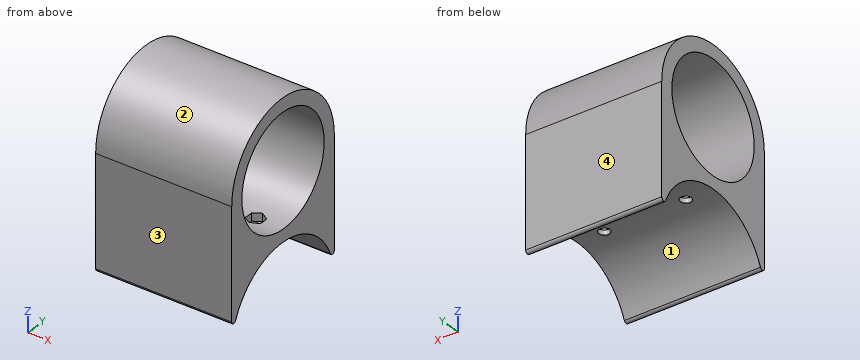
```python
from build123d import *

# Parameters (mm, degrees)
EXTRUDE_1_DEPTH      = 25
EXTRUDE_1_DEPTH_BACK = 25
SKETCH_1_R           = 20.25
SKETCH_2_R           = 2
CUT_EXTRUDE_1_DEPTH  = 41
CUT_EXTRUDE_2_DEPTH  = 3


with BuildPart() as part:
    # 草图1 → 凸台-拉伸1 (new, two sides: drawn at the far end of the back side and taken through both)
    with BuildSketch(Plane(origin=(0, 0, 0), x_dir=(0, 0, -1), z_dir=(1, 0, 0)).offset(-EXTRUDE_1_DEPTH_BACK)):
        with BuildLine():
            Line((39.950124379, 25.25), (0, 25.25))
            ThreePointArc((0, 25.25), (-25.25, 0), (0, -25.25))
            Line((0, -25.25), (39.950124379, -25.25))
            ThreePointArc((39.950124379, -25.25), (40.930891814, -24.445180015), (40.332976783, -23.326190476))
            ThreePointArc((40.332976783, -23.326190476), (24.75, 0), (40.332976783, 23.326190476))
            ThreePointArc((40.332976783, 23.326190476), (40.930891814, 24.445180015), (39.950124379, 25.25))
        make_face()
        Circle(SKETCH_1_R, mode=Mode.SUBTRACT)
    extrude(amount=EXTRUDE_1_DEPTH + EXTRUDE_1_DEPTH_BACK)

    # 草图2 → 切除-拉伸1 (cut)
    with BuildSketch(Plane.XY):
        with Locations((-15, 0)):
            Circle(SKETCH_2_R)
        with Locations((15, 0)):
            Circle(SKETCH_2_R)
    extrude(amount=-CUT_EXTRUDE_1_DEPTH, mode=Mode.SUBTRACT)

    # 草图3 → 切除-拉伸2 (cut)
    with BuildSketch(Plane.XY.offset(-20)):
        Polygon((-15, 3.25), (-17.814582562, 1.625), (-17.814582562, -1.625), (-15, -3.25), (-12.185417438, -1.625), (-12.185417438, 1.625), align=None)
        Polygon((15, 3.25), (12.185417438, 1.625), (12.185417438, -1.625), (15, -3.25), (17.814582562, -1.625), (17.814582562, 1.625), align=None)
    extrude(amount=-CUT_EXTRUDE_2_DEPTH, mode=Mode.SUBTRACT)


solid = part.part
```
Verification items for the finished model (mm, model axes). Face numbers are marked on the shaded views. Round coordinates to 2 decimals unless told otherwise and drop trailing zeros. Order: outer loops, then holes, each group sorted by start corner. A loop starts at its lowest first (then second) coordinate and runs counter-clockwise, first axis right, second up. Notation, with made-up numbers: (11.5, 16) - (48.5, 16) arc R22 ccw to (48.5, 46) - close; hole circle Ø6 at (17.5, 48.25). An arc over 180 degrees is marked (long way). Use CSV: the item, a comma, the result in double quotes.
(1) Thickness scan on probe 1 along X at (y, z) = (0, -23.45); probe 2 along Y at (x, z) = (-15, -24); probe 3 along Y at (x, z) = (13, 0). Record the ranges inside material, lowest first. Write a range as from..to.
Entries:
probe 1,"-25..-17, -13..13, 17..25"
probe 2,"-25.25..-2, 2..25.25"
probe 3,"-25.25..-20.25, 20.25..25.25"
(2) Section check B-B on y = 0. Record the boundary of the cut face in (x, z).
Entries:
outline,"(-25, -24.75) - (-17, -24.75) - (-17, -23) - (-17.81, -23) - (-17.81, -20.25) - (-25, -20.25) - close; (-25, 20.25) - (25, 20.25) - (25, 25.25) - (-25, 25.25) - close; (-13, -24.75) - (13, -24.75) - (13, -23) - (12.19, -23) - (12.19, -20.25) - (-12.19, -20.25) - (-12.19, -23) - (-13, -23) - close; (17, -24.75) - (25, -24.75) - (25, -20.25) - (17.81, -20.25) - (17.81, -23) - (17, -23) - close"
(3) Section check D-D on y = 11. Record the boundary of the cut face in (x, z).
Entries:
outline,"(-25, -27.27) - (25, -27.27) - (25, -17) - (-25, -17) - close; (-25, 17) - (25, 17) - (25, 22.73) - (-25, 22.73) - close"
(4) Gauge pin test, flat ends, axial feed: pin 1 Ø1.5 at (x, y) = (-4.5, -17.5) entering from +Z; pin 2 Ø3 at (x, y) = (-15, 0.5) entering from +Z; pin 3 Ø3 at (x, y) = (15.5, 19.5) entering from +Z. Record the tip position at first contact, or that the pin passes through.
Entries:
pin 1,"z = 18.89"
pin 2,"z = 25.25"
pin 3,"z = 17.71"
(5) Mould release check, pull along Y, two halves, no side actions. Record for the marked faces 1, 2, 3 and 4: released by +Y, released by -Y, zero draft, split by the parting line, or undercut.
Entries:
face 1,"undercut"
face 2,"split by the parting line"
face 3,"released by -Y"
face 4,"released by +Y"
(6) Section check C-C on z = 5.5. Record the boundary of the cut face in (x, y), and give its area (3 significant figures).
Entries:
outline,"(-25, -24.64) - (25, -24.64) - (25, -19.49) - (-25, -19.49) - close; (-25, 19.49) - (25, 19.49) - (25, 24.64) - (-25, 24.64) - close"
area,"515 mm^2"
(7) Section check A-A on x = -9.5. Record the boundary of the cut face in (y, z).
Entries:
outline,"(-25.25, -39.95) arc R1 ccw to (-23.33, -40.33) arc R25.25 cw to (23.33, -40.33) arc R1 ccw to (25.25, -39.95) - (25.25, 0) arc R25.25 ccw to (-25.25, 0) - close; hole circle Ø40.5 at (0, 0)"
